```python
from build123d import *

# Parameters (mm, degrees)
SKETCH_1_W          = 20
SKETCH_1_H          = 20
SKETCH_1_W_2        = 17
SKETCH_1_H_2        = 17
EXTRUDE_1_DEPTH     = 56
SKETCH_3_R          = 2.05
CUT_EXTRUDE_1_DEPTH = 23
SKETCH_4_R          = 2.05
CUT_EXTRUDE_2_DEPTH = 23


with BuildPart() as part:
    # 草图1 → 凸台-拉伸1 (new body)
    with BuildSketch(Plane.XY):
        Rectangle(SKETCH_1_W, SKETCH_1_H)
        Rectangle(SKETCH_1_W_2, SKETCH_1_H_2, mode=Mode.SUBTRACT)
    extrude(amount=EXTRUDE_1_DEPTH)

    # 草图3 → 切除-拉伸1 (cut)
    with BuildSketch(Plane.ZY.offset(10)):
        with Locations(Location((5, 0, 0), (0, 0, 270))):
            Circle(SKETCH_3_R)
        with Locations(Location((23, 0, 0), (0, 0, 270))):
            Circle(SKETCH_3_R)
    extrude(amount=-CUT_EXTRUDE_1_DEPTH, mode=Mode.SUBTRACT)

    # 草图4 → 切除-拉伸2 (cut)
    with BuildSketch(Plane(origin=(0, 10, 0), x_dir=(1, 0, 0), z_dir=(0, 1, 0))):
        with Locations(Location((0, -16, 0), (0, 0, 270))):
            Circle(SKETCH_4_R)
        with Locations(Location((0, -31, 0), (0, 0, 270))):
            Circle(SKETCH_4_R)
    extrude(amount=-CUT_EXTRUDE_2_DEPTH, mode=Mode.SUBTRACT)


solid = part.part
```
Work out the finished part from the listing and answer in its coordinate system (mm). A direction names the side the tool comes from. Round coordinates to 2 decimals unless told otherwise and drop trailing zeros. Write each loop counter-clockwise with the first axis right and the second up, starting at its lowest first coordinate (ties: lowest second). Pieces come first, ordered by that corner, then holes. Notation, with made-up numbers: (-10.75, -21) -> (37.25, -21) arc R14 ccw to (37.25, -4) -> close; hole circle Ø11 at (31, 15). An arc over 180 degrees is marked (long way). Write each question's results on one line, items separated by ' | '.
1) The part is cut by section A-A (z = 5). Write down the section's boundary in (x, y), and give its area (3 significant figures).
Findings:
outline: (-10, -10) -> (10, -10) -> (10, -2.05) -> (8.5, -2.05) -> (8.5, -8.5) -> (-8.5, -8.5) -> (-8.5, -2.05) -> (-10, -2.05) -> close; (-10, 2.05) -> (-8.5, 2.05) -> (-8.5, 8.5) -> (8.5, 8.5) -> (8.5, 2.05) -> (10, 2.05) -> (10, 10) -> (-10, 10) -> close | area: 98.7 mm²
2) Which of the six approach directions +Z, -Z, +X, -X, +Y, -Y give full straight-line access (tool end or side, diameter ignored) to faces 4 (the cylindrical face through (9.24, -0.946, 3.181)), 5 (the flat face through (0, -8.5, 28))?
Findings:
face 4: +X, -X | face 5: +Z, -Z
3) The part is cut by section D-D (y = 0). Write down the section's boundary in (x, z).
Findings:
outline: (-10, 0) -> (-8.5, 0) -> (-8.5, 2.95) -> (-10, 2.95) -> close; (-10, 7.05) -> (-8.5, 7.05) -> (-8.5, 20.95) -> (-10, 20.95) -> close; (-10, 25.05) -> (-8.5, 25.05) -> (-8.5, 56) -> (-10, 56) -> close; (8.5, 0) -> (10, 0) -> (10, 2.95) -> (8.5, 2.95) -> close; (8.5, 7.05) -> (10, 7.05) -> (10, 20.95) -> (8.5, 20.95) -> close; (8.5, 25.05) -> (10, 25.05) -> (10, 56) -> (8.5, 56) -> close
4) The part is cut by section C-C (x = 7.5). Write down the section's boundary in (y, z).
Findings:
outline: (-10, 0) -> (-8.5, 0) -> (-8.5, 56) -> (-10, 56) -> close; (8.5, 0) -> (10, 0) -> (10, 56) -> (8.5, 56) -> close
5) For a pull along X with two mould halves and no side action, classify faces 1 (the flat face through (-10, 0, 28)), 2 (the flat face through (-8.5, 0, 28)), 3 (the cylindrical face through (9.2, 1.5, 24.4)) as +X half, -X half, draft (parallel to the pull), parting line (faces both ways), or undercut.
Findings:
face 1: -X half | face 2: undercut | face 3: draft
6) Consider line 1 along X through (y, z) = (-2, 27.5); line 2 along Z through (x, y) = (9.25, 0). Determine where each line is inside the solid, lowest interval first. Write a range as [from, to].
Findings:
line 1: x = [-10, -8.5], [8.5, 10] | line 2: z = [0, 2.95], [7.05, 20.95], [25.05, 56]
7) The part is cut by section B-B (x = 0). Write down the section's boundary in (y, z), and give its area (3 significant figures).
Findings:
outline: (-10, 0) -> (-8.5, 0) -> (-8.5, 13.95) -> (-10, 13.95) -> close; (-10, 18.05) -> (-8.5, 18.05) -> (-8.5, 28.95) -> (-10, 28.95) -> close; (-10, 33.05) -> (-8.5, 33.05) -> (-8.5, 56) -> (-10, 56) -> close; (8.5, 0) -> (10, 0) -> (10, 13.95) -> (8.5, 13.95) -> close; (8.5, 18.05) -> (10, 18.05) -> (10, 28.95) -> (8.5, 28.95) -> close; (8.5, 33.05) -> (10, 33.05) -> (10, 56) -> (8.5, 56) -> close | area: 143 mm²
